```python
from build123d import *

# Parameters (mm, degrees)
F0_W      = 28.448
F0_H      = 73.406
F1_DEPTH  = 26.924
F2_W      = 104.648
F2_H      = 15.748
F3_DEPTH  = 28.575
F4_W      = 28.575
F4_H      = 104.648
F5_DEPTH  = 15.748
F6_W      = 4.826
F6_H      = 4.826
F5_FACE_W = 104.648
F5_FACE_H = 15.748
F7_DEPTH  = 28.575
F8_W      = 4.826
F8_H      = 4.826
F9_DEPTH  = 28.575
F11_DEPTH = 25.4
F13_DEPTH = 25.4
F15_DEPTH = 17.526
F17_DEPTH = 25.4
F18_W     = 35.052
F18_H     = 4.826
F18_H_2   = 15.748
F19_DEPTH = 17.526
F21_DEPTH = 25.4
F23_DEPTH = 25.4


with BuildPart() as f1:
    # F0 (on Top) → F1 (new body)
    with BuildSketch(Plane.XY):
        with Locations((0, -5.180504173)):
            Rectangle(F0_W, F0_H)
    extrude(amount=F1_DEPTH)

    # F2 (on face) → F3 (join)
    with BuildSketch(Plane.YZ.offset(14.224)):
        with Locations((10.440495827, 13.462)):
            Rectangle(F2_W, F2_H)
    extrude(amount=F3_DEPTH)

    # F4 (on face) → F5 (join)
    with BuildSketch(Plane.XY.offset(21.336)):
        with Locations((28.5115, 10.440495827)):
            Rectangle(F4_W, F4_H)
        with Locations((-28.5115, 10.440495827)):
            Rectangle(F4_W, F4_H)
    extrude(amount=-F5_DEPTH)

    # F6 (on face) + F5_face (on face) → F7 (cut)
    with BuildSketch(Plane.YZ.offset(42.799)):
        with Locations((-39.470504173, 8.001)):
            Rectangle(F6_W, F6_H)
    with BuildSketch(Plane(origin=(-42.799, 10.440495827, 13.462), x_dir=(0, -1, 0), z_dir=(-1, 0, 0))):
        Rectangle(F5_FACE_W, F5_FACE_H)
    extrude(amount=-F7_DEPTH, dir=(1, 0, 0), mode=Mode.SUBTRACT)

    # F8 (on face) → F9 (cut)
    with BuildSketch(Plane(origin=(-42.799, 0, 0), x_dir=(0, -1, 0), z_dir=(-1, 0, 0))):
        with Locations((39.470504173, 8.001)):
            Rectangle(F8_W, F8_H)
    extrude(amount=-F9_DEPTH, mode=Mode.SUBTRACT)

    # F10 (on face) → F11 (cut)
    with BuildSketch(Plane(origin=(0, 0, 5.588), x_dir=(1, 0, 0), z_dir=(0, 0, -1))):
        Polygon((-14.224, -34.189495827), (-42.799, -62.764495827), (-14.224, -62.764495827), align=None)
    extrude(amount=-F11_DEPTH, mode=Mode.SUBTRACT)

    # F12 (on face) → F13 (cut)
    with BuildSketch(Plane.XY.offset(21.336)):
        Polygon((42.799, 62.764495827), (14.224, 62.764495827), (14.224, 34.189495827), align=None)
    extrude(amount=-F13_DEPTH, mode=Mode.SUBTRACT)

    # F14 (on face) → F15 (join)
    with BuildSketch(Plane(origin=(-42.799, 0, 0), x_dir=(0, -1, 0), z_dir=(-1, 0, 0))):
        Polygon((-62.764495827, 26.162), (-62.764495827, 21.336), (-62.764495827, 5.588), (-62.764495827, 0.762), (-27.712495827, 0.762), (-27.712495827, 5.588), (-27.712495827, 21.336), (-27.712495827, 26.162), align=None)
    extrude(amount=-F15_DEPTH)

    # F16 (on face) → F17 (cut)
    with BuildSketch(Plane.XY.offset(26.162)):
        Polygon((-25.273, 45.238495827), (-25.273, 62.764495827), (-42.799, 62.764495827), align=None)
    extrude(amount=-F17_DEPTH, mode=Mode.SUBTRACT)

    # F18 (on face) → F19 (join)
    with BuildSketch(Plane.YZ.offset(42.799)):
        with Locations((45.238495827, 23.749)):
            Rectangle(F18_W, F18_H)
        with Locations((45.238495827, 13.462)):
            Rectangle(F18_W, F18_H_2)
        with Locations((45.238495827, 3.175)):
            Rectangle(F18_W, F18_H)
    extrude(amount=-F19_DEPTH)

    # F20 (on face) → F21 (cut)
    with BuildSketch(Plane.XY.offset(26.162)):
        Polygon((25.273, 45.238495827), (42.799, 62.764495827), (25.273, 62.764495827), align=None)
    extrude(amount=-F21_DEPTH, mode=Mode.SUBTRACT)

    # F22 (on face) → F23 (cut)
    with BuildSketch(Plane.XY.offset(21.336)):
        with BuildLine():
            ThreePointArc((-22.8882461797, 11.710495827), (-28.4762461797, 17.298495827), (-34.0642461797, 11.710495827))
            Line((-34.0642461797, 11.710495827), (-34.0642461797, -11.657504173))
            ThreePointArc((-34.0642461797, -11.657504173), (-28.4762461797, -17.245504173), (-22.8882461797, -11.657504173))
            Line((-22.8882461797, -11.657504173), (-22.8882461797, 11.710495827))
        make_face()
        with BuildLine():
            Line((34.0642461797, -11.657504173), (34.0642461797, 11.710495827))
            ThreePointArc((34.0642461797, 11.710495827), (28.4762461797, 17.298495827), (22.8882461797, 11.710495827))
            Line((22.8882461797, 11.710495827), (22.8882461797, -11.657504173))
            ThreePointArc((22.8882461797, -11.657504173), (28.4762461797, -17.245504173), (34.0642461797, -11.657504173))
        make_face()
    extrude(amount=-F23_DEPTH, mode=Mode.SUBTRACT)


solid = f1.part
```
Read the model definition and answer for the solid it produces. Units are mm, in the model's axes. A direction names the side the tool comes from. Coordinates: 2 decimals unless noted, no trailing zeros. Write each loop counter-clockwise with the first axis right and the second up, starting at its lowest first coordinate (ties: lowest second). Pieces come first, ordered by that corner, then holes. Notation, with made-up numbers: (23.5, -4.5) -> (68.5, -4.5) arc R26 cw to (68.5, 16.5) -> close; hole circle Ø6 at (37, -9.5). An arc over 180 degrees is marked (long way). Return JSON: item names as keys, results as strings.
1. A cutting plane is placed at D-D (x = -24). Determine the outline of the cut face in (y, z), and give its area (3 significant figures).
Found:
{"outline": "(-41.88, 10.41) -> (-37.06, 10.41) -> (-37.06, 5.59) -> (-15, 5.59) -> (-15, 21.34) -> (-41.88, 21.34) -> close; (15.06, 5.59) -> (43.97, 5.59) -> (43.97, 21.34) -> (15.06, 21.34) -> close", "area": "855 mm2"}
2. A cutting plane is placed at B-B (z = 23.5). Determine the outline of the cut face in (x, y), and give its area (3 significant figures).
Found:
{"outline": "(-42.8, 27.71) -> (-25.27, 27.71) -> (-25.27, 45.24) -> (-42.8, 62.76) -> close; (-14.22, -41.88) -> (14.22, -41.88) -> (14.22, 31.52) -> (-14.22, 31.52) -> close; (25.27, 27.71) -> (42.8, 27.71) -> (42.8, 62.76) -> (25.27, 45.24) -> close", "area": "3,010 mm2"}
3. A cutting plane is placed at A-A (y = 0.5). Determine the outline of the cut face in (x, z).
Found:
{"outline": "(-42.8, 5.59) -> (-34.06, 5.59) -> (-34.06, 21.34) -> (-42.8, 21.34) -> close; (-22.89, 5.59) -> (-14.22, 5.59) -> (-14.22, 0) -> (14.22, 0) -> (14.22, 5.59) -> (22.89, 5.59) -> (22.89, 21.34) -> (14.22, 21.34) -> (14.22, 26.92) -> (-14.22, 26.92) -> (-14.22, 21.34) -> (-22.89, 21.34) -> close; (34.06, 5.59) -> (42.8, 5.59) -> (42.8, 21.34) -> (34.06, 21.34) -> close"}
4. Find the intervals of material crossed by line 1 along X through (y, z) = (-7.5, 9.5); line 2 along Z through (x, y) = (-20.5, 25); line 3 along X through (y, z) = (-28, 24.5), in increasing order. Write a range as from..to.
Found:
{"line 1": "-42.8..-34.06, -22.89..22.89, 34.06..42.8", "line 2": "5.59..21.34", "line 3": "-14.22..14.22"}
5. A tool of negligible diameter and unlimited length cuts with its end or side. For faces 4 (the face through (25.273, 36, 24)), 5 (the face through (-29, -39, 10.414)), 6 (the face through (-34, 42, 0.762)), from which of +Z, -Z, +X, -X, +Y, -Y can it reach the whole face along a straight path? Write none if from no direction.
Found:
{"face 4": "+Z, +Y, -Y", "face 5": "-Z, -X, -Y", "face 6": "-Z, -X, +Y, -Y"}
6. Each of these flat-tipped pins is pushed along its axis until it touches: P1, Ø3, axis at y = -17.5, z = 23.5, coming from the -X side; P2, Ø4, axis at x = -35.5, z = 3.5, coming from the -Y side; P3, Ø14.5, axis at x = 30, y = -17.5, coming from the +Z side. Where does it stop, or does it pass through?
Found:
{"P1": "x = -14.22", "P2": "y = 27.71", "P3": "z = 21.34"}
7. Determine the mould class of faces 1 (the face through (34, 41, 0.762)), 2 (the face through (-25.273, 37, 24)), 3 (the face through (-42.799, 23, 14)) for opening direction X: pulls with the +X half, pulls with the -X half, needs draft (parallel to the pull), parting line crosses it, or undercut.
Found:
{"face 1": "needs draft", "face 2": "undercut", "face 3": "pulls with the -X half"}
8. A cutting plane is placed at C-C (z = 17). Determine the outline of the cut face in (x, y), and give its area (3 significant figures).
Found:
{"outline": "(-42.8, -41.88) -> (42.8, -41.88) -> (42.8, 62.76) -> (14.22, 34.19) -> (14.22, 31.52) -> (-14.22, 31.52) -> (-14.22, 34.19) -> (-42.8, 62.76) -> close; hole (-34.06, -11.66) arc R5.59 ccw to (-22.89, -11.66) -> (-22.89, 11.71) arc R5.59 ccw to (-34.06, 11.71) -> close; hole (22.89, -11.66) arc R5.59 ccw to (34.06, -11.66) -> (34.06, 11.71) arc R5.59 ccw to (22.89, 11.71) -> close", "area": "6,530 mm2"}
